```python
from build123d import *

# Parameters (mm, degrees)
IZIM1_W                     = 80
IZIM1_H                     = 14
Y_KSEKLIK_EKSTR_ZYON1_DEPTH = 20
KES_EKSTR_ZYON1_DEPTH       = 8
RADYUS1_R                   = 2


with BuildPart() as part:
    # Çizim1 → Yükseklik-Ekstrüzyon1 (new body)
    with BuildSketch(Plane.XY):
        with Locations((-11.444268973, 48.50560342)):
            Rectangle(IZIM1_W, IZIM1_H)
    extrude(amount=Y_KSEKLIK_EKSTR_ZYON1_DEPTH)

    # Çizim2 → Kes-Ekstrüzyon1 (cut)
    with BuildSketch(Plane.XY.offset(20)):
        Polygon((-11.444268973, 41.50560342), (-43.444268973, 41.50560342), (-43.444268973, 47.50560342), (20.555731027, 47.50560342), (20.555731027, 41.50560342), align=None)
    extrude(amount=-KES_EKSTR_ZYON1_DEPTH, mode=Mode.SUBTRACT)

    # Radyus1
    radyus1_edges = [part.edges().sort_by_distance(p)[0] for p in [
        (28.555731027, 48.50560342, 20),
        (-51.444268973, 48.50560342, 20),
        (28.555731027, 48.50560342, 0),
        (-51.444268973, 48.50560342, 0),
    ]]
    fillet(radyus1_edges, radius=RADYUS1_R)


solid = part.part
```
Work out the finished part from the listing and answer in its coordinate system (mm). A direction names the side the tool comes from. Give positions to 0.01 mm unless a question says otherwise; leave off trailing zeros. Loops run counter-clockwise (first coordinate to the right, second up) from the corner with the lowest first, then second, coordinate; pieces in that order, holes last. Notation, with made-up numbers: (-30.75, 26.5) -> (-6.75, 26.5) arc R22 cw to (-6.75, 65.5) -> close; hole circle Ø5 at (9.5, -23.75). An arc over 180 degrees is marked (long way). Write item = value, one per line. Start each with the question number.
(1) The mould has two halves that part along X. Classify faces 3 (the flat face through (28.556, 48, 10)), 4 (the flat face through (-11, 45, 12)), 5 (the flat face through (-12, 49, 0)): +X half, -X half, draft (parallel to the pull), parting line (faces both ways), or undercut.
(2) Given pin 1 Ø1.5 at (x, z) = (-28.5, 13) entering from -Y; pin 2 Ø1.8 at (x, y) = (-13, 45) entering from +Z, each flat-ended and moving along its own axis, determine where each tip first touches the part or whether it passes through.
(3) Find the intervals of material crossed by probe 1 along X at (y, z) = (42.5, 12.25); probe 2 along Y at (x, z) = (-23.5, 17); probe 3 along Z at (x, y) = (7, 46.5), in increasing order. Write a range as from..to.
(4) Which of the six approach directions +Z, -Z, +X, -X, +Y, -Y give full straight-line access (tool end or side, diameter ignored) to faces 1 (the flat face through (-51.444, 48, 10)), 2 (the flat face through (-43.444, 44, 16))?
(5) Find section C-C on y = 42.75. Give the vertices of the cut face in (x, z).
(6) Find section A-A on z = 13.25. Give the vertices of the cut face in (x, y).
(7) Find section B-B on x = 8. Give the vertices of the cut face in (y, z).
From the geometry:
q1.face_3 = +X half
q1.face_4 = undercut
q1.face_5 = draft
q2.pin_1 = 47.51
q2.pin_2 = 12
q3.probe_1 = -51.44..-43.44, 20.56..28.56
q3.probe_2 = 47.51..55.51
q3.probe_3 = 0..12
q4.face_1 = +Z, -Z, -X, +Y, -Y
q4.face_2 = +Z, -Y
q5.outline = (-51.44, 2) arc R2 ccw to (-49.44, 0) -> (26.56, 0) arc R2 ccw to (28.56, 2) -> (28.56, 18) arc R2 ccw to (26.56, 20) -> (20.56, 20) -> (20.56, 12) -> (-43.44, 12) -> (-43.44, 20) -> (-49.44, 20) arc R2 ccw to (-51.44, 18) -> close
q6.outline = (-51.44, 41.51) -> (-43.44, 41.51) -> (-43.44, 47.51) -> (20.56, 47.51) -> (20.56, 41.51) -> (28.56, 41.51) -> (28.56, 55.51) -> (-51.44, 55.51) -> close
q7.outline = (41.51, 0) -> (55.51, 0) -> (55.51, 20) -> (47.51, 20) -> (47.51, 12) -> (41.51, 12) -> close
